Can you work these out from the model? Positions are in its coordinate system, mm. A direction names the side the tool comes from. Give positions to 0.01 mm unless a question says otherwise; leave off trailing zeros. Loops run counter-clockwise (first coordinate to the right, second up) from the corner with the lowest first, then second, coordinate; pieces in that order, holes last. Notation, with made-up numbers: M 22,-32 L 30,-32 A23 ccw 30,-16 Z; hole C 44,33.5 d11. An arc over 180 degrees is marked long. One line per item, written item: value. Start each with the question number.
Autodesk Inventor part; units mm, degrees
ref_plane "YZ Plane" through (0, 0, 0) normal (1, 0, 0) x (0, 1, 0)
ref_plane "XZ Plane" through (0, 0, 0) normal (0, 1, 0) x (-1, 0, 0)
ref_plane "XY Plane" through (0, 0, 0) normal (0, 0, 1) x (1, 0, 0)
sketch "Sketch1" plane through (0, 0, 0) normal (0, 0, 1) x (1, 0, 0)
  line L0 (-17.78, 0) -> (17.78, 0)
  line L1 (0, -17.78) -> (0, 17.78)
  line L2 (-12.7, 12.7) -> (12.7, 12.7)
  line L3 (12.7, 12.7) -> (12.7, -12.7)
  line L4 (12.7, -12.7) -> (-12.7, -12.7)
  line L5 (-12.7, -12.7) -> (-12.7, 12.7)
  line L6 (9.525, 9.525) -> (-9.525, 9.525)
  line L7 (-9.525, 9.525) -> (-9.525, -9.525)
  line L8 (-9.525, -9.525) -> (9.525, -9.525)
  line L9 (9.525, -9.525) -> (9.525, 9.525)
  point P0 (0, 0)
  point P1 (-12.7, 0)
  point P2 (0, 12.7)
  dimension "d0" = 25.4
  dimension "d1" = 3.175
extrude "Extrusion1" add sketch "Sketch1" along normal mid plane 254 contours L5 L2 L1 L6 L7 L0 | L0 L7 L8 L1 L4 L5 | L1 L8 L9 L0 L3 L4 | L2 L3 L0 L9 L6 L1
sketch "Sketch3" plane through (-12.7, 12.7, 127) normal (0, 1, 0) x (1, 0, 0)
  line L0 (0, 0) -> (25.4, 0)
  line L1 (25.4, 0) -> (25.4, 254)
  line L2 (0, 0) -> (25.4, 14.6647)
  line L3 (0, 0) -> (25.4, 0)
  line L4 (25.4, 14.6647) -> (25.4, 0)
  point P0 (12.7, 127)
  dimension "d7" = 30
extrude "Extrusion3" cut sketch "Sketch3" against normal through all
sketch "Sketch4" plane through (-12.7, 12.7, -127) normal (0, 1, 0) x (1, 0, 0)
  line L0 (25.4, -239.3353) -> (25.4, 0)
  line L1 (25.4, 0) -> (0, 0)
  line L2 (0, 0) -> (25.4, -14.6647)
  line L3 (25.4, 0) -> (25.4, -14.6647)
  line L4 (25.4, 0) -> (0, 0)
  point P0 (12.7, -127)
  dimension "d10" = 30
extrude "Extrusion4" cut sketch "Sketch4" against normal through all
properties part number "tubing_template_0.125" material "Aluminum-6061"
Q1. Which directions (+Z, -Z, +X, -X, +Y, -Y) give clear straight access to the entire face, cutting with the end or side of a thin tool? Please do faces 4 (the face through (-0.18, -11.11, -119.77)), 5 (the face through (0, 9.525, -2)).
Q2. I need wall thicknesses on line 1 along Y through (x, z) = (1, -58.5) (3 decimals); line 2 along X through (y, z) = (-3.25, -116) (3 decimals). Which ranges of each line are inside material? Lowest first, please.
Q3. If we section it at B-B, the plane z = -100: Write out the boundary of the cut face in (x, y) (3 decimals).
Q4. If we section it at A-A, the plane y = -5.25: Write out the boundary of the cut face in (x, z) (3 decimals), plus the area to 3 significant figures.
Q5. For P1, Ø3, axis at x = 4, y = -9, coming from the +Z side; P2, Ø12, axis at x = -5, y = 4, coming from the -Z side; P3, Ø1.5, axis at x = 10, y = 9.5, coming from the -Z side, each with a flat end and sliding along its axis, tell me the tip position at first contact or that it passes through.
Q6. If we section it at C-C, the plane x = 6.75: Write out the boundary of the cut face in (y, z) (3 decimals).
Q7. If we mould it in two halves opening along Y, with no side actions, what happens to faces 1 (the face through (12.7, 0, -2)), 2 (the face through (0, -12.7, -2)), 3 (the face through (9.525, 0, -2))? For each: released by +Y, released by -Y, zero draft, split by the parting line, or undercut.
Response:
1. face 4: -Z, +X, +Y, -Y
1. face 5: +Z, -Z
2. line 1: -12.7 to -9.525, 9.525 to 12.7
2. line 2: -12.7 to -9.525
3. outline: M -12.7,-12.7 L 12.7,-12.7 L 12.7,12.7 L -12.7,12.7 Z; hole M -9.525,-9.525 L 9.525,-9.525 L 9.525,9.525 L -9.525,9.525 Z
4. outline: M -12.7,-127 L -9.525,-125.167 L -9.525,125.167 L -12.7,127 Z; M 9.525,-114.168 L 12.7,-112.335 L 12.7,112.335 L 9.525,114.168 Z
4. area: 1,520 mm^2
5. P1: z = 118.17
5. P2: z = -126.02
5. P3: z = -114.33
6. outline: M -12.7,-115.771 L -9.525,-115.771 L -9.525,115.771 L -12.7,115.771 Z; M 9.525,-115.771 L 12.7,-115.771 L 12.7,115.771 L 9.525,115.771 Z
7. face 1: zero draft
7. face 2: released by -Y
7. face 3: undercut
